from build123d import *

# Parameters (mm, degrees)
POCKET_DEPTH       = 146.174962
POLARPATTERN_COUNT = 3
SKETCH002_W        = 65
SKETCH002_H        = 20
SKETCH002_R        = 5
PAD_DEPTH          = 8
FILLET_R           = 3
FILLET001_R        = 1


with BuildPart() as part:
    # Sketch → Revolution (revolve)
    with BuildSketch(Plane.XZ):
        Polygon((2.75, 40), (11, 40), (11, 0), (10, -1), (10, -20), (6.014154, -20), (2.75, -13), align=None)
    revolve(axis=Axis((0, 0, 0), (0, 0, 1)))

    # Sketch001 (on DatumPlane) → Pocket (cut, through all)
    with BuildSketch(Plane(origin=(0, 0, -20), x_dir=(1, 0, 0), z_dir=(0, 1, 0))):
        with BuildLine():
            Line((0.5, -15), (0.5, 20))
            Line((0.5, 20), (-0.5, 20))
            Line((-0.5, 20), (-0.5, -15))
            ThreePointArc((-0.5, -15), (0, -15.5), (0.5, -15))
        make_face()
    pocket = extrude(amount=-POCKET_DEPTH, mode=Mode.SUBTRACT)

    # PolarPattern: Pocket ×3 about axis
    polarpattern_axis = Axis((0, 0, 0), (0, 0, 1))
    for i in range(1, POLARPATTERN_COUNT):
        add(pocket.rotate(polarpattern_axis, i * 360 / POLARPATTERN_COUNT), mode=Mode.SUBTRACT)

    # Sketch002 (on DatumPlane) → Pad (join)
    with BuildSketch(Plane.YZ.offset(11)):
        with Locations((0, 20)):
            Rectangle(SKETCH002_W, SKETCH002_H)
        with Locations((-20, 20)):
            Circle(SKETCH002_R, mode=Mode.SUBTRACT)
        with Locations((20, 20)):
            Circle(SKETCH002_R, mode=Mode.SUBTRACT)
    extrude(amount=-PAD_DEPTH)

    # Fillet
    fillet_edges = [part.edges().sort_by_distance(p)[0] for p in [
        (3, -32.5, 20),
        (3, 32.5, 20),
    ]]
    fillet(fillet_edges, radius=FILLET_R)

    # Fillet001
    fillet001_edges = [part.edges().sort_by_distance(p)[0] for p in [
        (3, 20.041503, 30),
        (3, 20.041503, 10),
        (3, -20.041503, 10),
        (3, -20.041503, 30),
    ]]
    fillet(fillet001_edges, radius=FILLET001_R)


solid = part.part
Read the model definition and answer for the solid it produces. Units are mm, in the model's axes. A direction names the side the tool comes from. Coordinates: 2 decimals unless noted, no trailing zeros. Loops run counter-clockwise (first coordinate to the right, second up) from the corner with the lowest first, then second, coordinate; pieces in that order, holes last.
Q1. Each of these flat-tipped pins is pushed along its axis until it touches: pin 1 Ø3.5 at (y, z) = (-7.5, -12.5) entering from -X; pin 2 Ø5.5 at (x, y) = (7.5, -19.5) entering from +Z; pin 3 Ø12 at (x, z) = (-4.5, 31.5) entering from +Y; pin 4 Ø9 at (y, z) = (20, 20) entering from -X. Where does it stop, or does it pass through?
Q2. Consider probe 1 along Y at (x, z) = (0, 2); probe 2 along Z at (x, y) = (8.5, 20); probe 3 along Y at (x, z) = (4, 20.5). Determine where each line is inside the solid, lowest interval first.
Q3. Which of the six approach directions +Z, -Z, +X, -X, +Y, -Y give full straight-line access (tool end or side, diameter ignored) to faces 4 (the face through (-5.701, 2.714, -12.395)), 5 (the face through (8, -19, 30)), 6 (the face through (7.06, -21.08, 15.12))?
Q4. The part is cut by section B-B on y = 20. Write down the section's boundary in (x, z).
Q5. The mould has two halves that part along Y. Classify faces 1 (the face through (9, -32.5, 20)), 2 (the face through (-2.17, -9.76, -10.63)), 3 (the face through (-0.596, -2.685, 13.871)): +Y half, -Y half, draft (parallel to the pull), parting line (faces both ways), or undercut.
Q6. The part is cut by section D-D on y = -21.5. Write down the section's boundary in (x, z).
Q7. The part is cut by section C-C on z = -6. Write down the section's boundary in (x, y), and give its area (3 significant figures).
Q8. The part is cut by section A-A on z = 20. Write down the section's boundary in (x, y).
Results below:
1. pin 1: stops at x = -8.18
1. pin 2: stops at z = 30
1. pin 3: stops at y = 11
1. pin 4: passes through
2. probe 1: y = -11 to -2.75, 2.75 to 11
2. probe 2: z = 10 to 15, 25 to 30
2. probe 3: y = -31.74 to -24.97, -15.03 to 15.03, 24.97 to 31.74
3. face 4: -Z
3. face 5: +Z, +X, -Y
3. face 6: +X, -X
4. outline: (3, 11) arc R1 ccw to (4, 10) - (11, 10) - (11, 15) - (3, 15) - close; (3, 25) - (11, 25) - (11, 30) - (4, 30) arc R1 ccw to (3, 29) - close
5. face 1: -Y half
5. face 2: parting line
5. face 3: undercut
6. outline: (3, 11) arc R1 ccw to (4, 10) - (11, 10) - (11, 15.23) - (3, 15.23) - close; (3, 24.77) - (11, 24.77) - (11, 30) - (4, 30) arc R1 ccw to (3, 29) - close
7. outline: (-8.9, 4.56) arc R10 ccw to (-0.5, -9.99) - (-0.5, -2.7) arc R2.75 cw to (-2.59, 0.92) - close; (-8.4, 5.43) - (-2.09, 1.79) arc R2.75 cw to (2.09, 1.79) - (8.4, 5.43) arc R10 ccw to start; (0.5, -9.99) arc R10 ccw to (8.9, 4.56) - (2.59, 0.92) arc R2.75 cw to (0.5, -2.7) - close
7. area: 269 mm2
8. outline: (3, -29.5) arc R3 ccw to (6, -32.5) - (11, -32.5) - (11, -25) - (3, -25) - close; (3, -15) - (11, -15) - (11, 15) - (3, 15) - (3, 10.58) arc R11 ccw (long way) to (3, -10.58) - close; (3, 25) - (11, 25) - (11, 32.5) - (6, 32.5) arc R3 ccw to (3, 29.5) - close; hole circle Ø5.5 at (0, 0)
